Here's the drawing with two shaded views (mm, measured from the low corner). I have some questions. A direction names the side the tool comes from. Give positions to 0.01 mm unless a question says otherwise; leave off trailing zeros. Write each loop counter-clockwise with the first axis right and the second up, starting at its lowest first coordinate (ties: lowest second). Pieces come first, ordered by that corner, then holes. Notation, with made-up numbers: (24.5, -13.5) - (79.5, -13.5) arc R34 cw to (79.5, 22.5) - close; hole circle Ø2 at (70.5, -6.5). An arc over 180 degrees is marked (long way). Use one line per item in the form item = value.
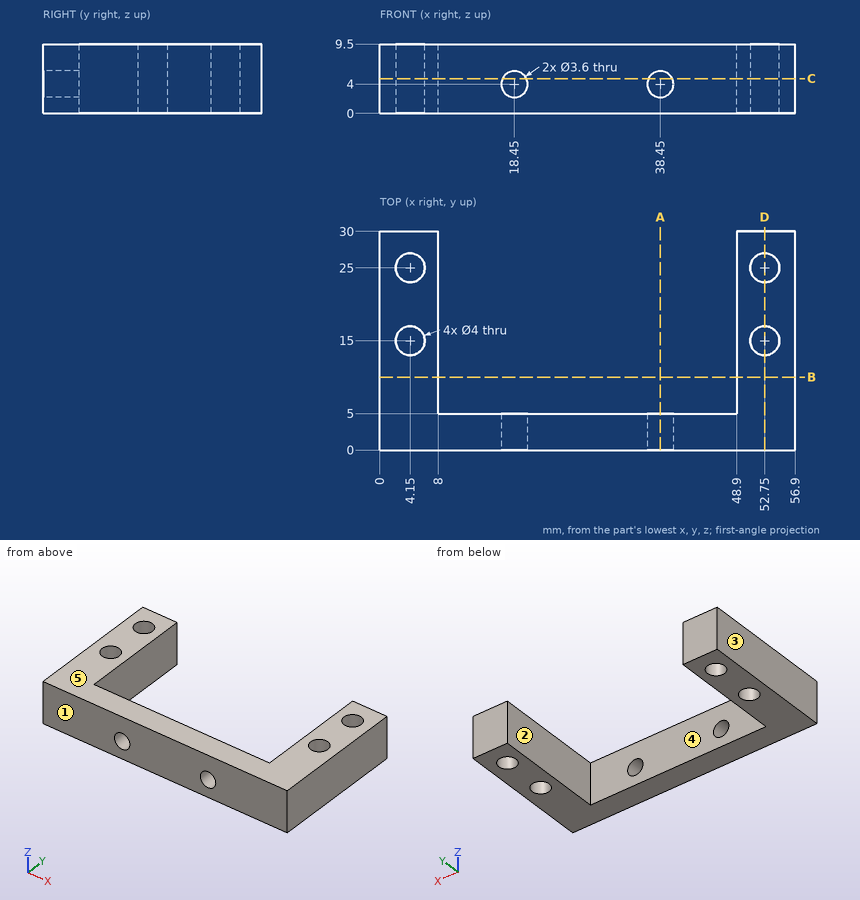
1. Imagine slicing it at C-C, the plane z = 4.75. List the corners of the cut face in (x, y) for me.
Response values:
outline = (0, 0) - (16.81, 0) - (16.81, 5) - (8, 5) - (8, 30) - (0, 30) - close; (20.09, 0) - (36.81, 0) - (36.81, 5) - (20.09, 5) - close; (40.09, 0) - (56.9, 0) - (56.9, 30) - (48.9, 30) - (48.9, 5) - (40.09, 5) - close; hole circle Ø4 at (4.15, 15); hole circle Ø4 at (4.15, 25); hole circle Ø4 at (52.75, 15); hole circle Ø4 at (52.75, 25)
2. For pin 1 (2 mm diameter, centred on x = 18.45, z = 4, fed in from -Y); pin 2 (5 mm diameter, centred on x = 32, z = 5, fed in from +Y), each with a flat end and sliding along its axis, tell me the tip position at first contact or that it passes through.
Response values:
pin_1 = through
pin_2 = 5
3. Which directions (+Z, -Z, +X, -X, +Y, -Y) give clear straight access to the entire face, cutting with the end or side of a thin tool? Please do the marked faces 1 and 2.
Response values:
face_1 = +Z, -Z, +X, -X, -Y
face_2 = +Z, -Z, +Y
4. Imagine slicing it at A-A, the plane x = 38.45. List the corners of the cut face in (y, z) for me, and give its area (3 significant figures).
Response values:
outline = (0, 0) - (5, 0) - (5, 2.2) - (0, 2.2) - close; (0, 5.8) - (5, 5.8) - (5, 9.5) - (0, 9.5) - close
area = 29.5 mm²
5. If we mould it in two halves opening along X, with no side actions, what happens to the marked faces 3, 4 and 5? For each: pulls with the +X half, pulls with the -X half, needs draft (parallel to the pull), parting line crosses it, or undercut.
Response values:
face_3 = pulls with the -X half
face_4 = undercut
face_5 = needs draft
6. Imagine slicing it at D-D, the plane x = 52.75. List the corners of the cut face in (y, z) for me.
Response values:
outline = (0, 0) - (13, 0) - (13, 9.5) - (0, 9.5) - close; (17, 0) - (23, 0) - (23, 9.5) - (17, 9.5) - close; (27, 0) - (30, 0) - (30, 9.5) - (27, 9.5) - close
7. If I drill on line 1 (X direction, y = 15, z = 7.5); line 2 (Y direction, x = 4.15, z = 4); line 3 (X direction, y = 18.75, z = 3), over which ranges is the centre line in solid material (lowest first)? Write a range as from..to.
Response values:
line_1 = 0..2.15, 6.15..8, 48.9..50.75, 54.75..56.9
line_2 = 0..13, 17..23, 27..30
line_3 = 0..8, 48.9..56.9
8. Imagine slicing it at B-B, the plane y = 10. List the corners of the cut face in (x, z) for me.
Response values:
outline = (0, 0) - (8, 0) - (8, 9.5) - (0, 9.5) - close; (48.9, 0) - (56.9, 0) - (56.9, 9.5) - (48.9, 9.5) - close
